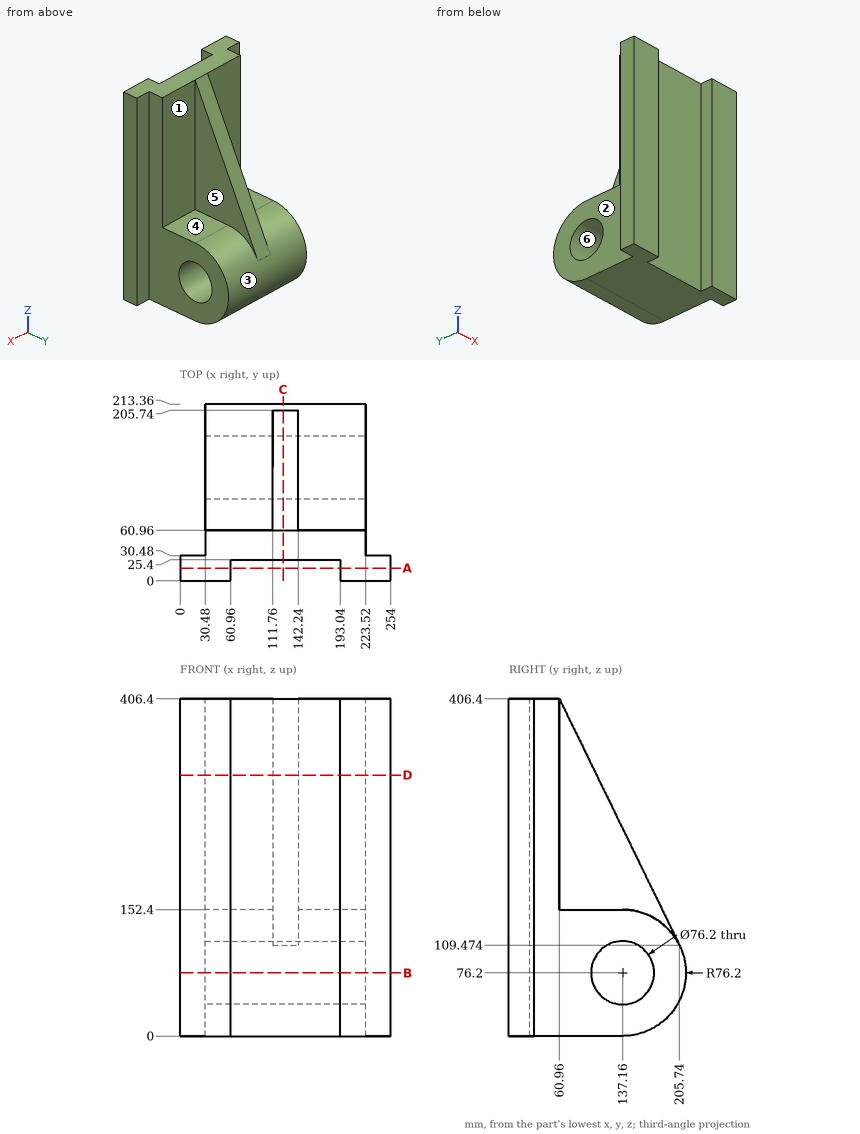
Input: dimensioned drawing with shaded views. Units: mm. Origin: part minimum x, y, z. A direction names the side the tool comes from. Round coordinates to 2 decimals unless told otherwise and drop trailing zeros. Write each loop counter-clockwise with the first axis right and the second up, starting at its lowest first coordinate (ties: lowest second). Pieces come first, ordered by that corner, then holes. Notation, with made-up numbers: (77.5, 29) -> (101.5, 29) arc R25 ccw to (101.5, 47) -> close; hole circle Ø9 at (-36, -21). An arc over 180 degrees is marked (long way). Use CSV: the item, a comma, the result in double quotes. Start each with the question number.
Q1. Section B-B (z = 76.2). Return loops of the section in (x, y).
Q2. Line query: L1, parallel to X at y = 9, z = 337; L2, parallel to Y at x = 132.5, z = 76.2; L3, parallel to Y at x = 60.5, z = 356. Output: solid intervals per line, ascending.
Q3. Pull-direction query (Z, two-part tool) for the marked faces 4, 5 and 6; classes: pulls with the +Z half, pulls with the -Z half, needs draft (parallel to the pull), parting line crosses it, or undercut.
Q4. Reachability of the marked faces 1, 2 and 3 from +Z, -Z, +X, -X, +Y, -Y: full face, straight path, thin tool, end or side. Return the list, or none.
Q5. Section D-D (z = 314.5). Return loops of the section in (x, y), plus the area to 3 significant figures.
Q6. Section A-A (y = 15.5). Return loops of the section in (x, z).
Q7. Section C-C (x = 124). Return loops of the section in (y, z), plus the area to 3 significant figures.
Q8. First-contact query: pin 1 Ø10 at (y, z) = (60.5, 323.5) entering from -X; pin 2 Ø4 at (x, y) = (68, 168.5) entering from -Z (3 decimals); pin 3 Ø1.5 at (x, y) = (215.5, 82.5) entering from +Z; pin 4 Ø12 at (x, y) = (96, 23) entering from +Z. Flat tips, straight axial feed; report the tip coordinate or a pass-through.
Result sheet:
1,outline,"(0, 0) -> (60.96, 0) -> (60.96, 25.4) -> (193.04, 25.4) -> (193.04, 0) -> (254, 0) -> (254, 30.48) -> (223.52, 30.48) -> (223.52, 99.06) -> (30.48, 99.06) -> (30.48, 30.48) -> (0, 30.48) -> close; (30.48, 175.26) -> (223.52, 175.26) -> (223.52, 213.36) -> (30.48, 213.36) -> close"
2,L1,"0 to 60.96, 193.04 to 254"
2,L2,"25.4 to 99.06, 175.26 to 213.36"
2,L3,"0 to 60.96"
3,face 4,"pulls with the +Z half"
3,face 5,"needs draft"
3,face 6,"undercut"
4,face 1,"+Z, +X, +Y"
4,face 2,"+Z, -Z, -X, +Y"
4,face 3,"+Y"
5,outline,"(0, 0) -> (60.96, 0) -> (60.96, 25.4) -> (193.04, 25.4) -> (193.04, 0) -> (254, 0) -> (254, 30.48) -> (223.52, 30.48) -> (223.52, 60.96) -> (142.24, 60.96) -> (142.24, 105.77) -> (111.76, 105.77) -> (111.76, 60.96) -> (30.48, 60.96) -> (30.48, 30.48) -> (0, 30.48) -> close"
5,area,"11,600 mm²"
6,outline,"(0, 0) -> (60.96, 0) -> (60.96, 406.4) -> (0, 406.4) -> close; (193.04, 0) -> (254, 0) -> (254, 406.4) -> (193.04, 406.4) -> close"
7,outline,"(25.4, 0) -> (137.16, 0) arc R76.2 ccw to (205.74, 109.41) -> (205.74, 109.47) -> (60.96, 406.4) -> (25.4, 406.4) -> close; hole circle Ø76.2 at (137.16, 76.2)"
7,area,"46,700 mm²"
8,pin 1,"x = 30.48"
8,pin 2,"z = 5.875"
8,pin 3,"z = 152.4"
8,pin 4,"z = 406.4"
